Could you check a few things on this drawing? It's one solid part, dimensions in mm from its lowest x, y, z. A direction names the side the tool comes from. Coordinates: 2 decimals unless noted, no trailing zeros. Write each loop counter-clockwise with the first axis right and the second up, starting at its lowest first coordinate (ties: lowest second). Pieces come first, ordered by that corner, then holes. Notation, with made-up numbers: M 7,62 L 49,62 A24 cw 49,93 Z; hole C 53.5,74.5 d4. An arc over 180 degrees is marked long. Use a Markdown table: item, result.
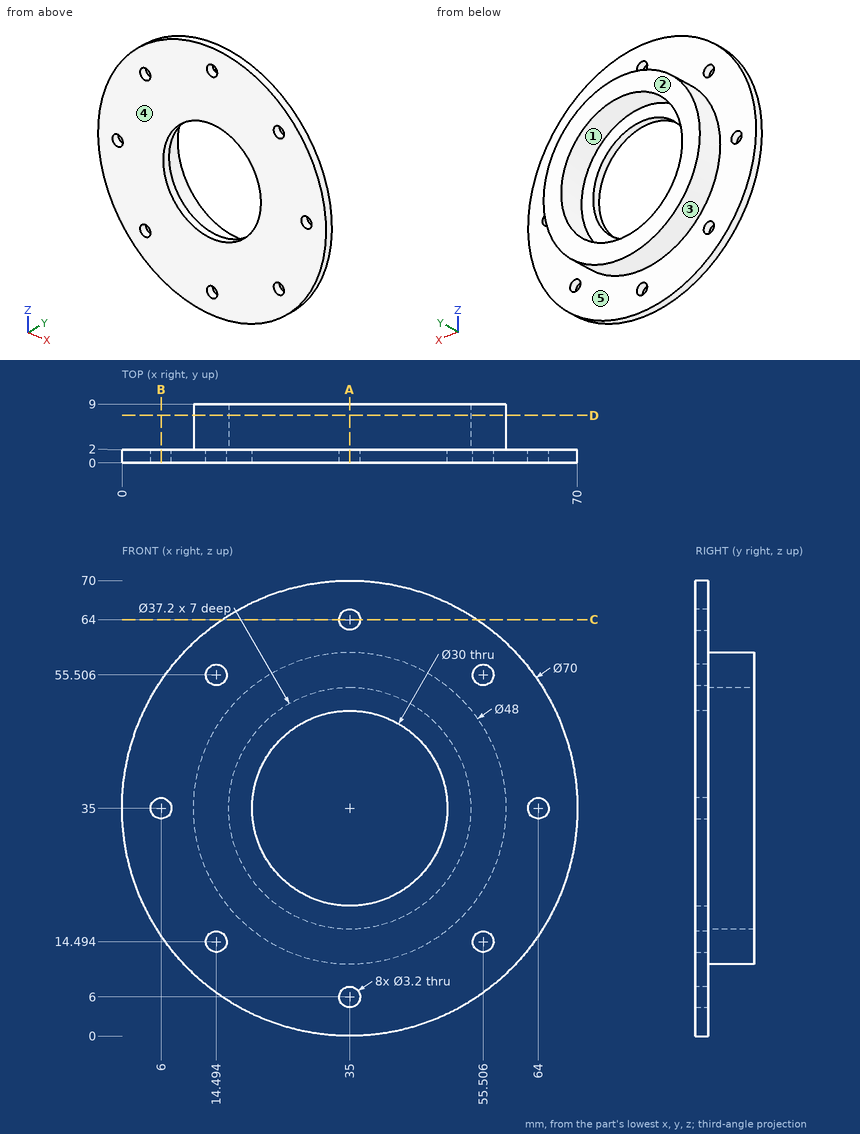
1. Will these pins go through, and if not, where does the flat tip stop? pin 1 Ø5 at (x, z) = (35, 6) entering from +Y; pin 2 Ø3 at (x, z) = (64, 35) entering from +Y; pin 3 Ø2 at (y, z) = (4, 32) entering from -X.
Answers follow:
| item | result |
|---|---|
| pin 1 | stops at y = 2 |
| pin 2 | passes through |
| pin 3 | stops at x = 11.08 |
2. Suppose I cut it at D-D on y = 7.25. Write out the boundary of the cut face in (x, z), and give its area (3 significant figures).
Answers follow:
| item | result |
|---|---|
| outline | C 35,35 d48; hole C 35,35 d37.2 |
| area | 723 mm2 |
3. Suppose I cut it at B-B on x = 6. Write out the boundary of the cut face in (y, z), and give its area (3 significant figures).
Answers follow:
| item | result |
|---|---|
| outline | M 0,15.4 L 2,15.4 L 2,33.4 L 0,33.4 Z; M 0,36.6 L 2,36.6 L 2,54.6 L 0,54.6 Z |
| area | 72.0 mm2 |
4. Suppose I cut it at A-A on x = 35. Write out the boundary of the cut face in (y, z).
Answers follow:
| item | result |
|---|---|
| outline | M 0,0 L 2,0 L 2,4.4 L 0,4.4 Z; M 0,7.6 L 2,7.6 L 2,11 L 9,11 L 9,16.4 L 2,16.4 L 2,20 L 0,20 Z; M 0,50 L 2,50 L 2,53.6 L 9,53.6 L 9,59 L 2,59 L 2,62.4 L 0,62.4 Z; M 0,65.6 L 2,65.6 L 2,70 L 0,70 Z |
5. I need wall thicknesses on probe 1 along X at (y, z) = (0.55, 35); probe 2 along X at (y, z) = (6.5, 35); probe 3 along Z at (x, y) = (56.5, 1.5). Which ranges of each line are inside material? Lowest first, please.
Answers follow:
| item | result |
|---|---|
| probe 1 | x = 0 to 4.4, 7.6 to 20, 50 to 62.4, 65.6 to 70 |
| probe 2 | x = 11 to 16.4, 53.6 to 59 |
| probe 3 | z = 7.38 to 13.24, 15.75 to 54.25, 56.76 to 62.62 |
6. Which directions (+Z, -Z, +X, -X, +Y, -Y) give clear straight access to the entire face, cutting with the end or side of a thin tool? Please do the marked faces 4 and 5.
Answers follow:
| item | result |
|---|---|
| face 4 | +Z, -Z, +X, -X, -Y |
| face 5 | +Y |
7. We'd pull the mould along X, two halves only. Please class the marked faces 1, 2 and 3: +X half, -X half, draft (parallel to the pull), parting line (faces both ways), or undercut.
Answers follow:
| item | result |
|---|---|
| face 1 | undercut |
| face 2 | draft |
| face 3 | parting line |
8. Suppose I cut it at C-C on z = 64. Write out the boundary of the cut face in (x, y).
Answers follow:
| item | result |
|---|---|
| outline | M 15.4,0 L 33.4,0 L 33.4,2 L 15.4,2 Z; M 36.6,0 L 54.6,0 L 54.6,2 L 36.6,2 Z |
